```python
from build123d import *

# Parameters (mm, degrees)
F0_R     = 8
F1_DEPTH = 20


with BuildPart() as f1:
    # F0 (on Front) → F1 (new body, symmetric)
    with BuildSketch(Plane.XZ):
        with BuildLine():
            Line((5.230114, 20.883032), (-30.769886, 20.883032))
            ThreePointArc((-30.769886, 20.883032), (-46.765878, 4.524912), (-30.053827, -11.100937))
            Line((-30.053827, -11.100937), (5.230114, -11.100937))
            Line((5.230114, -11.100937), (5.230114, -3.462973))
            Line((5.230114, -3.462973), (37.230114, -3.462973))
            Line((37.230114, -3.462973), (37.230114, 13.24507))
            Line((37.230114, 13.24507), (5.230114, 13.24507))
            Line((5.230114, 13.24507), (5.230114, 20.883032))
        make_face()
        with Locations((-30.769886, 4.883032)):
            Circle(F0_R, mode=Mode.SUBTRACT)
    extrude(amount=F1_DEPTH, both=True)


solid = f1.part
```
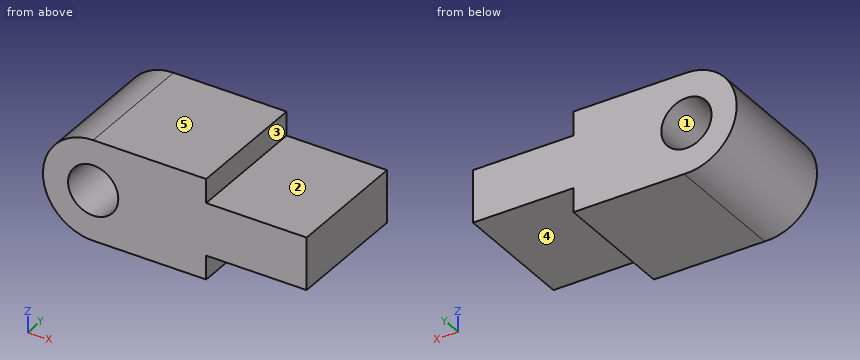
Geometry: final body of the model. Coordinates: model frame, mm. Face numbers are marked on the shaded views. A direction names the side the tool comes from. Round coordinates to 2 decimals unless told otherwise and drop trailing zeros. Loops run counter-clockwise (first coordinate to the right, second up) from the corner with the lowest first, then second, coordinate; pieces in that order, holes last. Notation, with made-up numbers: (63, 56) -> (122, 56) arc R26 cw to (122, 77) -> close; hole circle Ø10 at (-35.75, 44). An arc over 180 degrees is marked (long way). Use one line per item in the form item = value.
Item 1: Access query for the marked faces 4 and 5. Directions: +Z, -Z, +X, -X, +Y, -Y. A direction counts if a zero-diameter tool reaches every point of the face in a straight line with its end or side. Return the directions, or none.
Evaluation:
face_4 = -Z, +X, +Y, -Y
face_5 = +Z, +X, -X, +Y, -Y
Item 2: Contact query for flat-ended pins moving along their axis: pin 1 Ø2.5 at (y, z) = (1.5, -7.5) entering from +X; pin 2 Ø12 at (x, y) = (-19, 15.5) entering from -Z; pin 3 Ø13 at (x, z) = (-30.77, 4.88) entering from +Y; pin 4 Ø12 at (x, y) = (16.5, 5) entering from -Z. Output: stop coordinate, or through.
Evaluation:
pin_1 = 5.23
pin_2 = -11.1
pin_3 = through
pin_4 = -3.46
Item 3: Draft query along X for the marked faces 1, 2 and 3. Return one class per face: released by +X, released by -X, zero draft, split by the parting line, or undercut.
Evaluation:
face_1 = undercut
face_2 = zero draft
face_3 = released by +X
Item 4: Cut plane D-D on x = 11.5. Output: boundary loops of the cut face in (y, z), then the cut area to 3 significant figures.
Evaluation:
outline = (-20, -3.46) -> (20, -3.46) -> (20, 13.25) -> (-20, 13.25) -> close
area = 668 mm2
Item 5: Cut plane C-C on y = -5.5. Output: boundary loops of the cut face in (x, z).
Evaluation:
outline = (-30.77, 20.88) arc R16 ccw (long way) to (-30.05, -11.1) -> (5.23, -11.1) -> (5.23, -3.46) -> (37.23, -3.46) -> (37.23, 13.25) -> (5.23, 13.25) -> (5.23, 20.88) -> close; hole circle Ø16 at (-30.77, 4.88)
Item 6: Cut plane A-A on x = -37. Output: boundary loops of the cut face in (y, z), then the cut area to 3 significant figures.
Evaluation:
outline = (-20, -9.85) -> (20, -9.85) -> (20, -0.14) -> (-20, -0.14) -> close; (-20, 9.9) -> (20, 9.9) -> (20, 19.62) -> (-20, 19.62) -> close
area = 777 mm2
Item 7: Material intervals for probe 1 along Z at (x, y) = (-2, -10.5); probe 2 along Z at (x, y) = (16.5, -16.5); probe 3 along X at (y, z) = (-11, -2), sorted ascending.
Evaluation:
probe_1 = -11.1 to 20.88
probe_2 = -3.46 to 13.25
probe_3 = -45.21 to -34.85, -26.69 to 37.23
Item 8: Cut plane B-B on z = 8. Output: boundary loops of the cut face in (x, y).
Evaluation:
outline = (-46.46, -20) -> (-38.14, -20) -> (-38.14, 20) -> (-46.46, 20) -> close; (-23.4, -20) -> (37.23, -20) -> (37.23, 20) -> (-23.4, 20) -> close
